Input: part model. Units: mm. Frame: model coordinates. A direction names the side the tool comes from. Coordinates: 2 decimals unless noted, no trailing zeros. Write each loop counter-clockwise with the first axis right and the second up, starting at its lowest first coordinate (ties: lowest second). Pieces come first, ordered by that corner, then holes. Notation, with made-up numbers: (41, 9.5) - (82, 9.5) arc R28 ccw to (82, 43.5) - close; hole circle Ø10 at (-30, 68.5). An arc over 180 degrees is marked (long way). Use CSV: the item, a comma, the result in double quotes.
```python
from build123d import *

# Parameters (mm, degrees)
IZIM1_R                              = 59.2
Y_KSEKLIK_EKSTR_ZYON1_DEPTH          = 10
DAIRESEL_KAPLAMA1_COUNT              = 8
M8_HELISARMAL_I_IN_Z_VANA_MATKAB_2_D = 8.25


with BuildPart() as part:
    # Çizim1 → Yükseklik-Ekstrüzyon1 (new body)
    with BuildSketch(Plane.XY):
        Circle(IZIM1_R)
    extrude(amount=Y_KSEKLIK_EKSTR_ZYON1_DEPTH)

    # Çizim10 → M4x0.7 Helisarmal İçin Dişli Delik1 (revolve, cut)
    with BuildSketch(Plane(origin=(62, 0, 5), x_dir=(0, 0, -1), z_dir=(0, 1, 0))):
        Polygon((0, 0), (0, 17.2618073), (2.1, 16), (2.1, 0), align=None)
    m4x0_7_helisarmal_in_di_li_delik1 = revolve(axis=Axis((68.35, 0, 5), (-1, 0, 0)), mode=Mode.SUBTRACT)

    # Dairesel Kaplama1: M4x0.7 Helisarmal İçin Dişli Delik1 ×8 about axis
    dairesel_kaplama1_axis = Axis((0, 0, 10), (0, 0, -1))
    for i in range(1, DAIRESEL_KAPLAMA1_COUNT):
        add(m4x0_7_helisarmal_in_di_li_delik1.rotate(dairesel_kaplama1_axis, i * 360 / DAIRESEL_KAPLAMA1_COUNT), mode=Mode.SUBTRACT)

    # M8 Helisarmal için Zıvana matkabı2 (through all)
    with Locations(Plane(origin=(0, 0, 0), x_dir=(-1, 0, 0), z_dir=(0, 0, -1))):
        with Locations((0, 0)):
            Hole(M8_HELISARMAL_I_IN_Z_VANA_MATKAB_2_D / 2)


solid = part.part
```
(1) Draft query along Z for faces 5 (the cylindrical face through (-38.16, 36.36, 6.67)), 6 (the flat face through (-1, -12, 10)), 7 (the cylindrical face through (3.8, -1.6, 5.1)). Return one class per face: pulls with the +Z half, pulls with the -Z half, needs draft (parallel to the pull), parting line crosses it, or undercut.
Check values:
face 5,"undercut"
face 6,"pulls with the +Z half"
face 7,"needs draft"
(2) Pin query (flat end, axial travel): pin 1 Ø3 at (y, z) = (-43.5, 4.5) entering from +X; pin 2 Ø2.5 at (y, z) = (0, 5) entering from -X; pin 3 Ø5.5 at (x, z) = (0, 5) entering from +Y; pin 4 Ø4 at (y, z) = (-47.5, 5.5) entering from +X. Return the tip coordinate at first contact, or that it passes through.
Check values:
pin 1,"x = 41.03"
pin 2,"x = -45.49"
pin 3,"y = 59.2"
pin 4,"x = 37.87"
(3) Cut plane C-C on y = -37. State how many separate pieces and enclosed holes the cut face has, and give its area (3 significant figures).
Check values:
separate pieces,"1"
enclosed holes,"2"
area,"885 mm^2"
(4) Ray query, probe 1 along X at (y, z) = (-33, 6); probe 2 along Z at (x, y) = (0, 56); probe 3 along Y at (x, z) = (33.5, 4.25). Return the intervals inside material, ascending. Write a range as from..to.
Check values:
probe 1,"-49.15..-35.61, -31.51..31.51, 35.61..49.15"
probe 2,"0..2.9, 7.1..10"
probe 3,"-48.81..-36.27, -31.26..31.26, 36.27..48.81"
(5) Cut plane A-A on y = 49. Return loops of the section in (x, z), and give its area (3 significant figures).
Check values:
outline,"(-33.22, 0) - (33.22, 0) - (33.22, 10) - (-33.22, 10) - close; hole circle Ø4.2 at (0, 5)"
area,"651 mm^2"
(6) Cut plane B-B on x = 29.5. Return loops of the section in (y, z), and give its area (3 significant figures).
Check values:
outline,"(-51.33, 0) - (51.33, 0) - (51.33, 10) - (-51.33, 10) - close"
area,"1,030 mm^2"
(7) Reachability of faces 1 (the cylindrical face through (-52.69, -2.05, 5.46)), 2 (the cylindrical face through (-1.278, 52.693, 6.666)), 3 (the conical face through (32.04, -31.54, 5.08)), 4 (the cylindrical face through (-0.631, -52.693, 2.997)) from +Z, -Z, +X, -X, +Y, -Y: full face, straight path, thin tool, end or side. Return the list, or none.
Check values:
face 1,"-X"
face 2,"+Y"
face 3,"none"
face 4,"-Y"
(8) Cut plane D-D on y = 14.5. Return loops of the section in (x, z).
Check values:
outline,"(-57.4, 0) - (57.4, 0) - (57.4, 10) - (-57.4, 10) - close"
